```python
from build123d import *

# Parameters (mm, degrees)
SKETCH_1_R          = 9
EXTRUDE_1_DEPTH     = 5
CUT_EXTRUDE_1_DEPTH = 14.674794331
SKETCH_6_R          = 0.498388016
CUT_EXTRUDE_3_DEPTH = 50
EXTRUDE_START       = -0.5
SKETCH_3_R          = 14
SKETCH_3_R_2        = 9
EXTRUDE_2_DEPTH     = 0.5
SKETCH_5_R          = 14
SKETCH_5_R_2        = 9
EXTRUDE_3_DEPTH     = 0.5


with BuildPart() as part:
    # 草圖1 → 填料-伸長1 (new body)
    with BuildSketch(Plane(origin=(0, 0, 0), x_dir=(1, 0, 0), z_dir=(0, 1, 0))):
        with Locations(Location((0, 0, 0), (0, 0, 270))):
            Circle(SKETCH_1_R)
    extrude(amount=EXTRUDE_1_DEPTH)

    # 草圖2 → 除料-伸長1 (cut, through all)
    with BuildSketch(Plane(origin=(0, 5, 0), x_dir=(1, 0, 0), z_dir=(0, 1, 0))):
        with BuildLine():
            Line((-0.93, 1.264911064), (-0.93, -1.264911064))
            ThreePointArc((-0.93, -1.264911064), (0.708801806, -1.400892573), (1.57, 0))
            ThreePointArc((1.57, 0), (0.708801806, 1.400892573), (-0.93, 1.264911064))
        make_face()
    extrude(amount=-CUT_EXTRUDE_1_DEPTH, mode=Mode.SUBTRACT)

    # 草圖6 → 除料-伸長3 (cut, symmetric)
    with BuildSketch(Plane(origin=(0, 0, 0), x_dir=(0, 0, -1), z_dir=(1, 0, 0))):
        with Locations((-8.29743406, 2.581049417)):
            Circle(SKETCH_6_R)
    extrude(amount=CUT_EXTRUDE_3_DEPTH, both=True, mode=Mode.SUBTRACT)

    # 草圖3 → 填料-伸長2 (add)
    with BuildSketch(Plane(origin=(0, 5, 0), x_dir=(1, 0, 0), z_dir=(0, 1, 0)).offset(EXTRUDE_START)):
        with Locations(Location((0, 0, 0), (0, 0, 270))):
            Circle(SKETCH_3_R)
        with Locations(Location((0, 0, 0), (0, 0, 270))):
            Circle(SKETCH_3_R_2, mode=Mode.SUBTRACT)
    extrude(amount=EXTRUDE_2_DEPTH)

    # 草圖5 → 填料-伸長3 (add)
    with BuildSketch(Plane.XZ):
        with Locations(Location((0, 0, 0), (0, 0, 90))):
            Circle(SKETCH_5_R)
        with Locations(Location((0, 0, 0), (0, 0, 270))):
            Circle(SKETCH_5_R_2, mode=Mode.SUBTRACT)
    extrude(amount=-EXTRUDE_3_DEPTH)


solid = part.part
```
Input: part model. Units: mm. Frame: model coordinates. A direction names the side the tool comes from. Give positions to 0.01 mm unless a question says otherwise; leave off trailing zeros. Order: outer loops, then holes, each group sorted by start corner. A loop starts at its lowest first (then second) coordinate and runs counter-clockwise, first axis right, second up. Notation, with made-up numbers: M 88.5,37.5 L 120.5,37.5 A23 cw 120.5,69.5 Z; hole C -3.75,-39 d6. An arc over 180 degrees is marked long. Return JSON: item names as keys, results as strings.
1) Access query for faces 5 (the face through (-9, 4.5, 3)), 6 (the face through (0, 5, 3)), 7 (the face through (-0.93, 3, 0)). Directions: +Z, -Z, +X, -X, +Y, -Y. A direction counts if a zero-diameter tool reaches every point of the face in a straight line with its end or side. Return the directions, or none.
Taken from the geometry:
{"face 5": "none", "face 6": "+Z, -Z, +X, -X, +Y", "face 7": "+Y, -Y"}
2) Mould query, pull axis Y, two halves, no side actions, for faces 1 (the face through (-13.67, 4.75, -3.03)), 2 (the face through (0.06, 2.73, 7.82)), 3 (the face through (9, 0.5, 3)), 4 (the face through (0, 0, 3)). Classes: released by +Y, released by -Y, zero draft, split by the parting line, or undercut.
Taken from the geometry:
{"face 1": "zero draft", "face 2": "undercut", "face 3": "undercut", "face 4": "released by -Y"}
3) Contact query for flat-ended pins moving along their axis: pin 1 (1.5 mm diameter, centred on y = 3.5, z = -3.5, fed in from +X); pin 2 (2 mm diameter, centred on y = 2.5, z = 0.5, fed in from +X); pin 3 (1 mm diameter, centred on x = 2.5, y = 0.5, fed in from +Z). Output: stop coordinate, or through.
Taken from the geometry:
{"pin 1": "stops at x = 8.57", "pin 2": "stops at x = 9", "pin 3": "stops at z = 13.86"}
4) Line query: L1, parallel to Y at x = 4.5, z = -11; L2, parallel to X at y = 0.35, z = 0.25; L3, parallel to X at y = 2.95, z = 0.25. Output: solid intervals per line, ascending. Write a range as [from, to].
Taken from the geometry:
{"L1": "y = [0, 0.5], [4.5, 5]", "L2": "x = [-14, -0.93], [1.55, 14]", "L3": "x = [-9, -0.93], [1.55, 9]"}
5) Section query D-D on y = 1. Output: boundary loops of the cut face in (x, z).
Taken from the geometry:
{"outline": "C 0,0 d18; hole M -0.93,-1.26 A1.57 ccw long -0.93,1.26 Z"}
6) Section query A-A on x = 0. Output: boundary loops of the cut face in (y, z), and give its area (3 significant figures).
Taken from the geometry:
{"outline": "M 0,-14 L 0.5,-14 L 0.5,-9 L 4.5,-9 L 4.5,-14 L 5,-14 L 5,-1.57 L 0,-1.57 Z; M 0,1.57 L 5,1.57 L 5,14 L 4.5,14 L 4.5,9 L 0.5,9 L 0.5,14 L 0,14 Z; hole C 2.58,8.3 d1", "area": "83.5 mm2"}
7) Section query B-B on z = 0.5. Output: boundary loops of the cut face in (x, y).
Taken from the geometry:
{"outline": "M -13.99,0 L -0.93,0 L -0.93,5 L -13.99,5 L -13.99,4.5 L -8.99,4.5 L -8.99,0.5 L -13.99,0.5 Z; M 1.49,0 L 13.99,0 L 13.99,0.5 L 8.99,0.5 L 8.99,4.5 L 13.99,4.5 L 13.99,5 L 1.49,5 Z"}
8) Section query C-C on x = 11.75. Output: boundary loops of the cut face in (y, z).
Taken from the geometry:
{"outline": "M 0,-7.61 L 0.5,-7.61 L 0.5,7.61 L 0,7.61 Z; M 4.5,-7.61 L 5,-7.61 L 5,7.61 L 4.5,7.61 Z"}
